Design review of the part shown in the three views and the two pictorial views. Dimensions are in mm from the part's minimum x, y and z. A direction names the side the tool comes from. Coordinates: 2 decimals unless noted, no trailing zeros. Loops run counter-clockwise (first coordinate to the right, second up) from the corner with the lowest first, then second, coordinate; pieces in that order, holes last. Notation, with made-up numbers: (46.5, -4) -> (70.5, -4) arc R29 cw to (70.5, 28) -> close; hole circle Ø11 at (14, 45.25). An arc over 180 degrees is marked (long way). One line per item, written item: value. Start each with the question number.
1. Insertion check: pin 1 (3 mm diameter, centred on y = 146, z = 201.5, fed in from +X); pin 2 (4 mm diameter, centred on x = 11.5, z = 122.5, fed in from +Y); pin 3 (12 mm diameter, centred on x = 24, z = 131.5, fed in from -Y); pin 4 (4 mm diameter, centred on y = 128.5, z = 200.5, fed in from -X). Each pin has a flat end and moves straight along its axis. Give the tip position at first contact, or say it passes through.
2. Machinability: for the marked faces 1 and 2, which of the approach directions +Z, -Z, +X, -X, +Y, -Y give a long, thin tool a straight path to every point of the face, cutting with its end or side? Answer none if there is none.
3. For probe 1 along Z at (x, y) = (5, 120); probe 2 along Z at (x, y) = (26.5, 120); probe 3 along Y at (x, z) = (31, 120), list the stretches that pass through material, from the lowest coordinate up.
4. Add section C-C on x = 14.5. Write out the cut boundary in (y, z).
5. Add section D-D on y = 183.5. Write out the cut boundary in (x, z), plus the area to 3 significant figures.
6. Add section A-A on y = 120. Write out the cut boundary in (x, z).
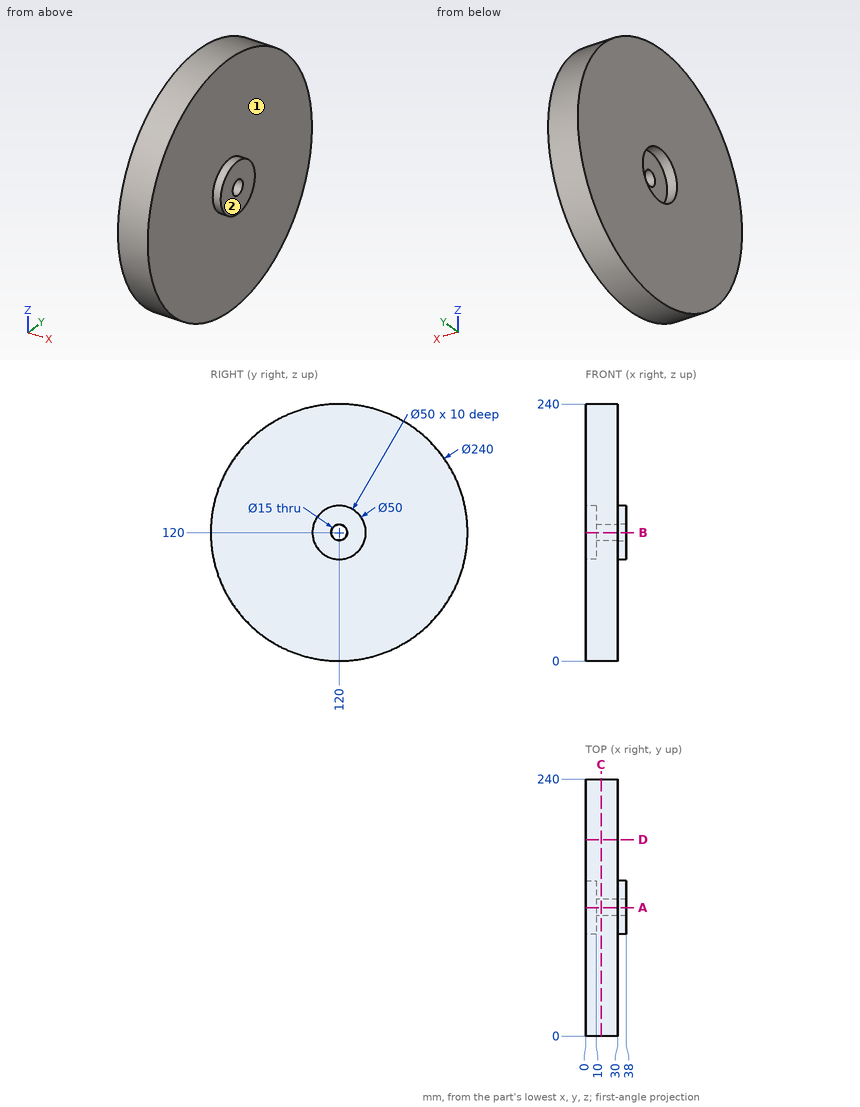
Worked answers:
1. pin 1: stops at x = 30
1. pin 2: stops at y = 240
1. pin 3: stops at y = 0.13
1. pin 4: stops at x = 0
2. face 1: +X
2. face 2: +Z, -Z, +X, +Y, -Y
3. probe 1: z = 0 to 95, 145 to 240
3. probe 2: z = 0 to 112.5, 127.5 to 240
3. probe 3: y = 95 to 112.5, 127.5 to 145
4. outline: circle Ø240 at (120, 120); hole circle Ø15 at (120, 120)
5. outline: (0, 18.18) -> (30, 18.18) -> (30, 221.82) -> (0, 221.82) -> close
5. area: 6,110 mm²
6. outline: (0, 0) -> (30, 0) -> (30, 95) -> (38, 95) -> (38, 112.5) -> (10, 112.5) -> (10, 95) -> (0, 95) -> close; (0, 145) -> (10, 145) -> (10, 127.5) -> (38, 127.5) -> (38, 145) -> (30, 145) -> (30, 240) -> (0, 240) -> close
